```python
from build123d import *

# Parameters (mm, degrees)
F0_W     = 88.9
F0_H     = 88.9
F1_DEPTH = 812.8
F2_W     = 38.1
F2_H     = 50.8
F3_DEPTH = 44.45
F4_W     = 12.7
F4_H     = 50.8
F5_DEPTH = 88.901


with BuildPart() as f1:
    # F0 (on Top) → F1 (new body)
    with BuildSketch(Plane.XY):
        Rectangle(F0_W, F0_H)
    extrude(amount=F1_DEPTH)

    # F2 (on face) → F3 (cut)
    with BuildSketch(Plane.YZ.offset(44.45)):
        with Locations((0, 768.35)):
            Rectangle(F2_W, F2_H)
        with Locations((0, 228.6)):
            Rectangle(F2_W, F2_H)
    extrude(amount=-F3_DEPTH, mode=Mode.SUBTRACT)

    # F4 (on face) → F5 (cut, through all)
    with BuildSketch(Plane.XZ.offset(44.45)):
        with Locations((0, 635)):
            Rectangle(F4_W, F4_H)
        with Locations((0, 330.2)):
            Rectangle(F4_W, F4_H)
    extrude(amount=-F5_DEPTH, mode=Mode.SUBTRACT)


solid = f1.part
```
Model file for the job. Use its own axes, mm. A direction names the side the tool comes from. Give positions to 0.01 mm unless a question says otherwise; leave off trailing zeros. Loops run counter-clockwise (first coordinate to the right, second up) from the corner with the lowest first, then second, coordinate; pieces in that order, holes last. Notation, with made-up numbers: M 11,20 L 41,20 A20 ccw 41,24 Z; hole C 49.5,-4 d3. An arc over 180 degrees is marked long. Use one line per item in the form item = value.
Item 1: Slice it at A-A on z = 316.5. List the corners of the cut face in (x, y).
Filled in:
outline = M -44.45,-44.45 L -6.35,-44.45 L -6.35,44.45 L -44.45,44.45 Z; M 6.35,-44.45 L 44.45,-44.45 L 44.45,44.45 L 6.35,44.45 Z
Item 2: Flat gauge pins, fed straight in: pin 1 Ø19 at (y, z) = (-9, 231) entering from +X; pin 2 Ø14 at (x, y) = (3, -10.5) entering from -Z. Where does each tip first touch, or does it go through?
Filled in:
pin_1 = 0
pin_2 = 0
Item 3: Slice it at C-C on x = 14.5. List the corners of the cut face in (y, z).
Filled in:
outline = M -44.45,0 L 44.45,0 L 44.45,812.8 L -44.45,812.8 Z; hole M -19.05,203.2 L 19.05,203.2 L 19.05,254 L -19.05,254 Z; hole M -19.05,742.95 L 19.05,742.95 L 19.05,793.75 L -19.05,793.75 Z
Item 4: Drill centre lines: L1, parallel to Z at x = -3, y = 2; L2, parallel to Z at x = 6.5, y = -9; L3, parallel to Y at x = 4.5, z = 220. Where is each one in solid material? Low to high.
Filled in:
L1 = 0 to 304.8, 355.6 to 609.6, 660.4 to 812.8
L2 = 0 to 203.2, 254 to 742.95, 793.75 to 812.8
L3 = -44.45 to -19.05, 19.05 to 44.45
Item 5: Slice it at B-B on y = 5. List the corners of the cut face in (x, z), and give its area (3 significant figures).
Filled in:
outline = M -44.45,0 L 44.45,0 L 44.45,203.2 L 0,203.2 L 0,254 L 44.45,254 L 44.45,742.95 L 0,742.95 L 0,793.75 L 44.45,793.75 L 44.45,812.8 L -44.45,812.8 Z; hole M -6.35,304.8 L 6.35,304.8 L 6.35,355.6 L -6.35,355.6 Z; hole M -6.35,609.6 L 6.35,609.6 L 6.35,660.4 L -6.35,660.4 Z
area = 66,500 mm^2
Item 6: Slice it at D-D on y = -37.5. List the corners of the cut face in (x, z), and give its area (3 significant figures).
Filled in:
outline = M -44.45,0 L 44.45,0 L 44.45,812.8 L -44.45,812.8 Z; hole M -6.35,304.8 L 6.35,304.8 L 6.35,355.6 L -6.35,355.6 Z; hole M -6.35,609.6 L 6.35,609.6 L 6.35,660.4 L -6.35,660.4 Z
area = 71,000 mm^2
Item 7: Two-plate mould, pull along Y, no slides. Class faces 4 (the flat face through (23, -19.05, 768)), 5 (the flat face through (-1, 44.45, 401)), 6 (the flat face through (-1, -44.45, 401)), 7 (the flat face through (0, -1, 355.6)): released by +Y, released by -Y, zero draft, split by the parting line, or undercut.
Filled in:
face_4 = undercut
face_5 = released by +Y
face_6 = released by -Y
face_7 = zero draft
Item 8: Which spindle directions (+Z, -Z, +X, -X, +Y, -Y) get a long thin tool onto all of the face, cutting with end or side? Do faces 1 (the flat face through (0, 0, 229)), 2 (the flat face through (44.45, -1, 401)), 3 (the flat face through (6.35, -1, 330)). Say none if no direction does.
Filled in:
face_1 = +X
face_2 = +Z, -Z, +X, +Y, -Y
face_3 = +Y, -Y
